```python
from build123d import *

# Parameters (mm, degrees)
F2_W     = 20
F2_H     = 18.99
F3_DEPTH = 28
F4_R     = 3
F5_R     = 1.75
F6_DEPTH = 25


with BuildPart() as f1:
    # F0 (on Top) → F1 (revolve)
    with BuildSketch(Plane.XY):
        Polygon((0, 30), (0, 0), (11, 0), (10, 30), align=None)
    revolve(axis=Axis((0, 15, 0), (0, 1, 0)))

    # F2 (on face) → F3 (cut, through all)
    with BuildSketch(Plane(origin=(0, 30, 0), x_dir=(-1, 0, 0), z_dir=(0, 1, 0))):
        with Locations((11.01, 10.505)):
            Rectangle(F2_W, F2_H)
        with Locations((-11.01, 10.505)):
            Rectangle(F2_W, F2_H)
        with Locations((11.01, -10.505)):
            Rectangle(F2_W, F2_H)
        with Locations((-11.01, -10.505)):
            Rectangle(F2_W, F2_H)
    extrude(amount=-F3_DEPTH, mode=Mode.SUBTRACT)

    # F4
    f4_edges = [f1.edges().sort_by_distance(p)[0] for p in [
        (9.987208, 30, 0.505647),
        (0, 30, 10),
        (-10, 30, 0),
        (0, 30, -10),
    ]]
    fillet(f4_edges, radius=F4_R)

    # F5 (on face) → F6 (cut)
    with BuildSketch(Plane(origin=(0, 2, 0), x_dir=(-1, 0, 0), z_dir=(0, 1, 0))):
        with Locations((-5.6568542495, 5.6568542495)):
            Circle(F5_R)
        with Locations((5.6568542495, -5.6568542495)):
            Circle(F5_R)
        with Locations((-5.6568542495, -5.6568542495)):
            Circle(F5_R)
        with Locations((5.6568542495, 5.6568542495)):
            Circle(F5_R)
    extrude(amount=-F6_DEPTH, mode=Mode.SUBTRACT)


solid = f1.part
```
Input: part model. Units: mm. Frame: model coordinates. A direction names the side the tool comes from. Round coordinates to 2 decimals unless told otherwise and drop trailing zeros. Write each loop counter-clockwise with the first axis right and the second up, starting at its lowest first coordinate (ties: lowest second). Pieces come first, ordered by that corner, then holes. Notation, with made-up numbers: (-30, 16) -> (18, 16) arc R11 ccw to (18, 37) -> close; hole circle Ø3 at (13.25, -20). An arc over 180 degrees is marked (long way). Answer as CSV lines item,"result".
1. Reachability of faces 1 (the flat face through (4.9, 2, 3.8)), 2 (the flat face through (-6, 16, 1.01)), 3 (the flat face through (-6, 16, -1.01)), 4 (the flat face through (6, 16, -1.01)) from +Z, -Z, +X, -X, +Y, -Y: full face, straight path, thin tool, end or side. Return the list, or none.
Geometry says:
face 1,"+Z, +X, +Y"
face 2,"+Z, -X, +Y"
face 3,"-Z, -X, +Y"
face 4,"-Z, +X, +Y"
2. Mould query, pull axis X, two halves, no side actions, for faces 5 (the cylindrical face through (-7.273, 1.014, 4.987)), 6 (the flat face through (1.01, 16, 6)), 7 (the flat face through (4.9, 2, -3.7)). Classes: +X half, -X half, draft (parallel to the pull), parting line (faces both ways), or undercut.
Geometry says:
face 5,"undercut"
face 6,"+X half"
face 7,"draft"
3. Contact query for flat-ended pins moving along their axis: P1, Ø5, axis at x = -7.5, y = 21.5, coming from the -Z side; P2, Ø3, axis at x = -7.5, z = -6, coming from the +Y side; P3, Ø2, axis at x = 5.66, z = 5.66, coming from the -Y side; P4, Ø5, axis at x = 8, y = 16.5, coming from the +Z side. Output: stop coordinate, or through.
Geometry says:
P1,"stops at z = -1.01"
P2,"stops at y = 2"
P3,"passes through"
P4,"stops at z = 1.01"
4. Section C-C (y = 2.5). Return the cut outline in (x, z).
Geometry says:
outline,"(-10.87, -1.01) -> (-1.01, -1.01) -> (-1.01, -10.87) arc R10.92 ccw to (1.01, -10.87) -> (1.01, -1.01) -> (10.87, -1.01) arc R10.92 ccw to (10.87, 1.01) -> (1.01, 1.01) -> (1.01, 10.87) arc R10.92 ccw to (-1.01, 10.87) -> (-1.01, 1.01) -> (-10.87, 1.01) arc R10.92 ccw to start"
5. Ray query, L1, parallel to X at y = 19, z = -4; L2, parallel to Y at x = -6, z = -1.75. Return the intervals inside material, ascending. Write a range as [from, to].
Geometry says:
L1,"x = [-1.01, 1.01]"
L2,"y = [0, 2]"
6. Section D-D (z = -4.75). Give the number of separate pieces and of enclosed holes in the cut face, plus the area to 3 significant figures.
Geometry says:
separate pieces,"3"
enclosed holes,"0"
area,"84.1 mm^2"
7. Section A-A (z = 0). Return the cut outline in (x, y), plus the area to 3 significant figures.
Geometry says:
outline,"(-11, 0) -> (11, 0) -> (10.1, 27.1) arc R3 ccw to (7.1, 30) -> (-7.1, 30) arc R3 ccw to (-10.1, 27.1) -> close"
area,"626 mm^2"
8. Section B-B (x = 0). Return the cut outline in (y, z).
Geometry says:
outline,"(0, -11) -> (27.1, -10.1) arc R3 ccw to (30, -7.1) -> (30, 7.1) arc R3 ccw to (27.1, 10.1) -> (0, 11) -> close"
